Here's how the part is built. I have some questions about the finished solid (model axes, mm). A direction names the side the tool comes from. Round coordinates to 2 decimals unless told otherwise and drop trailing zeros. Loops run counter-clockwise (first coordinate to the right, second up) from the corner with the lowest first, then second, coordinate; pieces in that order, holes last. Notation, with made-up numbers: M -0.75,-0.5 L 45.25,-0.5 A21 cw 45.25,38.5 Z; hole C 20.25,45.5 d9. An arc over 180 degrees is marked long. Use a Markdown table: item, result.
```python
from build123d import *

# Parameters (mm, degrees)
SKETCH_1_W          = 15
SKETCH_1_H          = 5
SKETCH_1_W_2        = 20
SKETCH_1_W_3        = 10
EXTRUDE_1_DEPTH     = 10
SKETCH_1_3_W        = 20
SKETCH_1_3_H        = 5
SKETCH_1_3_W_2      = 10
EXTRUDE_2_DEPTH     = 15
SKETCH_1_4_W        = 15
SKETCH_1_4_H        = 5
EXTRUDE_3_DEPTH     = 20
CUT_EXTRUDE_1_DEPTH = 20
SCALE_1_SCALE       = 0.2


with BuildPart() as part:
    # Sketch 1 → Extrude 1 (new body)
    with BuildSketch(Plane(origin=(0, 0, 0), x_dir=(1, 0, 0), z_dir=(0, 1, 0))):
        with Locations((-7.5, 7.5)):
            Rectangle(SKETCH_1_W, SKETCH_1_H)
        Polygon((15, -5), (15, 10), (0, 10), (0, 5), (-15, 5), (-15, -5), (5, -5), align=None)
        with Locations((-5, -7.5)):
            Rectangle(SKETCH_1_W_2, SKETCH_1_H)
        with Locations((10, -7.5)):
            Rectangle(SKETCH_1_W_3, SKETCH_1_H)
    extrude(amount=EXTRUDE_1_DEPTH)

    # Sketch 1_3 → Extrude 2 (add)
    with BuildSketch(Plane(origin=(0, 0, 0), x_dir=(1, 0, 0), z_dir=(0, 1, 0))):
        with Locations((-5, -7.5)):
            Rectangle(SKETCH_1_3_W, SKETCH_1_3_H)
        with Locations((10, -7.5)):
            Rectangle(SKETCH_1_3_W_2, SKETCH_1_3_H)
    extrude(amount=EXTRUDE_2_DEPTH)

    # Sketch 1_4 → Extrude 3 (add)
    with BuildSketch(Plane(origin=(0, 0, 0), x_dir=(1, 0, 0), z_dir=(0, 1, 0))):
        with Locations((-7.5, 7.5)):
            Rectangle(SKETCH_1_4_W, SKETCH_1_4_H)
    extrude(amount=EXTRUDE_3_DEPTH)

    # Sketch 2 → Cut-Extrude 1 (cut)
    with BuildSketch(Plane.XY.offset(10)):
        Polygon((5, 15), (15, 10), (15, 15), align=None)
    extrude(amount=-CUT_EXTRUDE_1_DEPTH, mode=Mode.SUBTRACT)


with BuildPart() as part_1:
    # Scale 1: scaled about (-0.960451977, 6.638418079, -0.127118644)
    add(part.part.scale(SCALE_1_SCALE).moved(Location((-0.768361582, 5.310734463, -0.101694915))))


solid = part_1.part
```
Q1. We'd pull the mould along Z, two halves only. Please class faces 1 (the flat face through (-1, 7.311, 0)), 2 (the flat face through (-1.8, 8.311, 1.4)), 3 (the flat face through (-1, 7, 1.898)), 4 (the flat face through (-2, 8, -1.102)): pulls with the +Z half, pulls with the -Z half, needs draft (parallel to the pull), parting line crosses it, or undercut.
Return value:
| item | result |
|---|---|
| face 1 | undercut |
| face 2 | needs draft |
| face 3 | pulls with the +Z half |
| face 4 | undercut |
Q2. Imagine slicing it at D-D, the plane y = 8. Please give me the cut outline in (x, z).
Return value:
| item | result |
|---|---|
| outline | M -3.77,-2.1 L -0.77,-2.1 L -0.77,-1.1 L -3.77,-1.1 Z; M -3.77,0.9 L 0.85,0.9 L 0.85,1.9 L -3.77,1.9 Z |
Q3. For faces 5 (the flat face through (-0.768, 8.3, -1.6)), 6 (the flat face through (-1, 8, 0.898)), 7 (the flat face through (-1, 5.311, 0)), which set-ups out of +Z, -Z, +X, -X, +Y, -Y let a thin tool reach every point of the face, with its end or its side?
Return value:
| item | result |
|---|---|
| face 5 | -Z, +X, +Y |
| face 6 | +X, -X, +Y |
| face 7 | +Z, -Z, +X, -X, -Y |
Q4. I need wall thicknesses on line 1 (Z direction, x = -2.25, y = 7.45); line 2 (Z direction, x = -0.5, y = 7.85); line 3 (Y direction, x = 0.5, z = 0.05). Which ranges of each line are inside material? Lowest first, please. Write a range as from..to.
Return value:
| item | result |
|---|---|
| line 1 | z = -2.1..-1.1, 0.9..1.9 |
| line 2 | z = 0.9..1.9 |
| line 3 | y = 5.31..7.31 |
Q5. Imagine slicing it at B-B, the plane x = -2.75. Please give me the cut outline in (y, z).
Return value:
| item | result |
|---|---|
| outline | M 5.31,-2.1 L 9.31,-2.1 L 9.31,-1.1 L 7.31,-1.1 L 7.31,0.9 L 8.31,0.9 L 8.31,1.9 L 5.31,1.9 Z |
Q6. Imagine slicing it at C-C, the plane z = 1.6. Please give me the cut outline in (x, y).
Return value:
| item | result |
|---|---|
| outline | M -3.77,5.31 L 2.23,5.31 L 2.23,7.31 L 0.23,8.31 L -3.77,8.31 Z |
Q7. Will these pins go through, and if not, where does the flat tip stop? P1, Ø0.8, axis at y = 8.5, z = -2, coming from the +X side; P2, Ø1.5, axis at x = 1.5, z = -1.5, coming from the +Y side; P3, Ø1.1, axis at x = -1.5, z = 1, coming from the +Y side.
Return value:
| item | result |
|---|---|
| P1 | stops at x = -0.77 |
| P2 | stops at y = 7.31 |
| P3 | stops at y = 8.31 |
Q8. Imagine slicing it at A-A, the plane y = 7.6. Please give me the cut outline in (x, z).
Return value:
| item | result |
|---|---|
| outline | M -3.77,-2.1 L -0.77,-2.1 L -0.77,-1.1 L -3.77,-1.1 Z; M -3.77,0.9 L 1.65,0.9 L 1.65,1.9 L -3.77,1.9 Z |
